```python
from build123d import *

# Parameters (mm, degrees)
BOSS_EXTRUDE1_DEPTH = 250
CUT_EXTRUDE3_DEPTH  = 10
BOSS_EXTRUDE2_DEPTH = 20
CUT_EXTRUDE4_START  = -240
CUT_EXTRUDE4_DEPTH  = 240
FILLET1_R           = 5
FILLET2_R           = 5


with BuildPart() as part:
    # Sketch1 → Boss-Extrude1 (new body)
    with BuildSketch(Plane(origin=(0, 0, 0), x_dir=(1, 0, 0), z_dir=(0, 1, 0))):
        with BuildLine():
            Line((-175, 110), (175, 110))
            ThreePointArc((175, 110), (189.142135624, 104.142135624), (195, 90))
            Line((195, 90), (195, -90))
            ThreePointArc((195, -90), (189.142135624, -104.142135624), (175, -110))
            Line((175, -110), (-175, -110))
            ThreePointArc((-175, -110), (-189.142135624, -104.142135624), (-195, -90))
            Line((-195, -90), (-195, 90))
            ThreePointArc((-195, 90), (-189.142135624, 104.142135624), (-175, 110))
        make_face()
    extrude(amount=BOSS_EXTRUDE1_DEPTH)

    # Sketch3 → Cut-Extrude3 (cut)
    with BuildSketch(Plane.XZ):
        with BuildLine():
            Line((0, -5.659305135), (-173.94856301, -97.886397626))
            ThreePointArc((-173.94856301, -97.886397626), (-169.597393146, -99.464428485), (-165, -100))
            Line((-165, -100), (165, -100))
            ThreePointArc((165, -100), (169.597393146, -99.464428485), (173.94856301, -97.886397626))
            Line((173.94856301, -97.886397626), (0, -5.659305135))
        make_face()
        with BuildLine():
            ThreePointArc((-185, -80), (-184.19844413, -85.605331658), (-181.8580257, -90.761364667))
            Line((-181.8580257, -90.761364667), (-10.673956744, 0))
            Line((-10.673956744, 0), (-181.8580257, 90.761364667))
            ThreePointArc((-181.8580257, 90.761364667), (-184.19844413, 85.605331658), (-185, 80))
            Line((-185, 80), (-185, -80))
        make_face()
        with BuildLine():
            Line((-173.94856301, 97.886397626), (0, 5.659305135))
            Line((0, 5.659305135), (173.94856301, 97.886397626))
            ThreePointArc((173.94856301, 97.886397626), (169.597393146, 99.464428485), (165, 100))
            Line((165, 100), (-165, 100))
            ThreePointArc((-165, 100), (-169.597393146, 99.464428485), (-173.94856301, 97.886397626))
        make_face()
        with BuildLine():
            Line((181.8580257, 90.761364667), (10.673956744, 0))
            Line((10.673956744, 0), (181.8580257, -90.761364667))
            ThreePointArc((181.8580257, -90.761364667), (184.19844413, -85.605331658), (185, -80))
            Line((185, -80), (185, 80))
            ThreePointArc((185, 80), (184.19844413, 85.605331658), (181.8580257, 90.761364667))
        make_face()
    extrude(amount=-CUT_EXTRUDE3_DEPTH, mode=Mode.SUBTRACT)

    # Sketch5 → Boss-Extrude2 (add)
    with BuildSketch(Plane(origin=(0, 250, 0), x_dir=(1, 0, 0), z_dir=(0, 1, 0))):
        with BuildLine():
            Line((195, 130), (-195, 130))
            ThreePointArc((-195, 130), (-209.142135624, 124.142135624), (-215, 110))
            Line((-215, 110), (-215, -110))
            ThreePointArc((-215, -110), (-209.142135624, -124.142135624), (-195, -130))
            Line((-195, -130), (195, -130))
            ThreePointArc((195, -130), (209.142135624, -124.142135624), (215, -110))
            Line((215, -110), (215, 110))
            ThreePointArc((215, 110), (209.142135624, 124.142135624), (195, 130))
        make_face()
    extrude(amount=BOSS_EXTRUDE2_DEPTH)

    # Sketch6 → Cut-Extrude4 (cut)
    with BuildSketch(Plane(origin=(0, 270, 0), x_dir=(1, 0, 0), z_dir=(0, 1, 0)).offset(CUT_EXTRUDE4_START)):
        with BuildLine():
            Line((-165, -100), (165, -100))
            ThreePointArc((165, -100), (179.142135624, -94.142135624), (185, -80))
            Line((185, -80), (185, 80))
            ThreePointArc((185, 80), (179.142135624, 94.142135624), (165, 100))
            Line((165, 100), (-165, 100))
            ThreePointArc((-165, 100), (-179.142135624, 94.142135624), (-185, 80))
            Line((-185, 80), (-185, -80))
            ThreePointArc((-185, -80), (-179.142135624, -94.142135624), (-165, -100))
        make_face()
    extrude(amount=CUT_EXTRUDE4_DEPTH, mode=Mode.SUBTRACT)

    # Fillet1
    fillet1_edges = [part.edges().sort_by_distance(p)[0] for p in [
        (179.142135624, 270, -94.142135624),
        (0, 270, -100),
        (-179.142135624, 270, -94.142135624),
        (-185, 270, 0),
        (-179.142135624, 270, 94.142135624),
        (0, 270, 100),
        (179.142135624, 270, 94.142135624),
        (185, 270, 0),
    ]]
    fillet(fillet1_edges, radius=FILLET1_R)

    # Fillet2
    fillet2_edges = [part.edges().sort_by_distance(p)[0] for p in [
        (-209.142135624, 270, 124.142135624),
        (0, 270, 130),
        (209.142135624, 270, 124.142135624),
        (215, 270, 0),
        (209.142135624, 270, -124.142135624),
        (0, 270, -130),
        (-209.142135624, 270, -124.142135624),
        (-215, 270, 0),
    ]]
    fillet(fillet2_edges, radius=FILLET2_R)


solid = part.part
```
Could you check a few things on this model? Use its own coordinates, in mm. A direction names the side the tool comes from. Coordinates: 2 decimals unless noted, no trailing zeros. Loops run counter-clockwise (first coordinate to the right, second up) from the corner with the lowest first, then second, coordinate; pieces in that order, holes last. Notation, with made-up numbers: M 52,78.5 L 92,78.5 A4 cw 92,85.5 Z; hole C -2,15.5 d6. An arc over 180 degrees is marked long. Put each result on its own line as item: value. Start each with the question number.
(1) Will these pins go through, and if not, where does the flat tip stop? P1, Ø5, axis at x = 111, z = 2, coming from the -Y side; P2, Ø2, axis at y = 43, z = -74.5, coming from the -X side; P3, Ø3, axis at y = 4.5, z = 37, coming from the +X side.
(2) I need wall thicknesses on line 1 (X direction, y = 256.5, z = -69); line 2 (X direction, y = 57, z = 52.5); line 3 (Z direction, x = 25, y = 159). Which ranges of each line are inside material? Lowest first, please. Write a range as from..to.
(3) Suppose I cut it at B-B on x = 115.5. Please give me the cut outline in (y, z), then the cut area to 3 significant figures.
(4) Thinking about a two-plate mould opening in Z: for faces 5 (the face through (2, 123, 110)), 6 (the face through (-97.464, 4.93, -46.016)), 7 (the face through (15, 270, -112)), which applies, pulls with the +Z half, pulls with the -Z half, needs draft (parallel to the pull), parting line crosses it, or undercut?
(5) For faces 1 (the face through (189.297, 123.25, 103.986)), 2 (the face through (-95.068, 4.93, 44.745)), 3 (the face through (-208.986, 257.395, -124.297)), 4 (the face through (179.297, 145.855, -93.986)), which set-ups out of +Z, -Z, +X, -X, +Y, -Y let a thin tool reach every point of the face, with its end or its side?
(6) Suppose I cut it at A-A on y = 95. Please give me the cut outline in (x, z).
(7) Suppose I cut it at C-C on z = 12. Please give me the cut outline in (x, y), then the cut area to 3 significant figures.
Solutions:
1. P1: stops at y = 10
1. P2: stops at x = -195
1. P3: stops at x = 195
2. line 1: x = -215..-185, 185..215
2. line 2: x = -195..-185, 185..195
2. line 3: z = -110..-100, 100..110
3. outline: M 0,-110 L 250,-110 L 250,-130 L 265,-130 A5 ccw 270,-125 L 270,-105 A5 ccw 265,-100 L 30,-100 L 30,100 L 265,100 A5 ccw 270,105 L 270,125 A5 ccw 265,130 L 250,130 L 250,110 L 0,110 L 0,100 L 10,100 L 10,66.9 L 0,66.9 L 0,55.58 L 10,55.58 L 10,-55.58 L 0,-55.58 L 0,-66.9 L 10,-66.9 L 10,-100 L 0,-100 Z
3. area: 10,400 mm2
4. face 5: pulls with the +Z half
4. face 6: undercut
4. face 7: needs draft
5. face 1: +Z, +X, -Y
5. face 2: -Y
5. face 3: -Z, -X, +Y, -Y
5. face 4: +Y
6. outline: M -195,-90 A20 ccw -175,-110 L 175,-110 A20 ccw 195,-90 L 195,90 A20 ccw 175,110 L -175,110 A20 ccw -195,90 Z; hole M -185,-80 A20 ccw -165,-100 L 165,-100 A20 ccw 185,-80 L 185,80 A20 ccw 165,100 L -165,100 A20 ccw -185,80 Z
7. outline: M -215,250 L -195,250 L -195,0 L -185,0 L -185,10 L -33.31,10 L -33.31,0 L -11.96,0 L -11.96,10 L 11.96,10 L 11.96,0 L 33.31,0 L 33.31,10 L 185,10 L 185,0 L 195,0 L 195,250 L 215,250 L 215,265 A5 ccw 210,270 L 190,270 A5 ccw 185,265 L 185,30 L -185,30 L -185,265 A5 ccw -190,270 L -210,270 A5 ccw -215,265 Z
7. area: 14,000 mm2
